The listing builds one solid part. Answer for the finished solid, in the listing's coordinates (mm). Face numbers are marked on the shaded views. Coordinates: 2 decimals unless noted, no trailing zeros. Write each loop counter-clockwise with the first axis right and the second up, starting at its lowest first coordinate (ties: lowest second). Pieces come first, ordered by that corner, then holes.
from build123d import *

# Parameters (mm, degrees)
CROQUIS1_W              = 7
CROQUIS1_H              = 18.3
SALIENTE_EXTRUIR1_DEPTH = 2.6
CORTAR_EXTRUIR2_DEPTH   = 10
REDONDEO1_R             = 1.5


with BuildPart() as part:
    # Croquis1 → Saliente-Extruir1 (new body)
    with BuildSketch(Plane(origin=(0, 0, 0), x_dir=(1, 0, 0), z_dir=(0, 1, 0))):
        Rectangle(CROQUIS1_W, CROQUIS1_H)
    extrude(amount=SALIENTE_EXTRUIR1_DEPTH)

    # Croquis2 → Cortar-Extruir2 (cut)
    with BuildSketch(Plane(origin=(0, 2.6, 0), x_dir=(1, 0, 0), z_dir=(0, 1, 0))):
        with BuildLine():
            ThreePointArc((3.25, 3.725), (3.426776695, 3.651776695), (3.5, 3.475))
            Line((3.5, 3.475), (3.5, 6.225))
            ThreePointArc((3.5, 6.225), (3.426776695, 6.048223305), (3.25, 5.975))
            Line((3.25, 5.975), (2.767072698, 5.975))
            ThreePointArc((2.767072698, 5.975), (2.651546276, 6.003293785), (2.562169292, 6.081770833))
            ThreePointArc((2.562169292, 6.081770833), (-1.35, 4.85), (2.562169292, 3.618229167))
            ThreePointArc((2.562169292, 3.618229167), (2.651546276, 3.696706215), (2.767072698, 3.725))
            Line((2.767072698, 3.725), (3.25, 3.725))
        make_face()
        with BuildLine():
            ThreePointArc((3.5, -3.475), (3.426776695, -3.651776695), (3.25, -3.725))
            Line((3.25, -3.725), (2.767072698, -3.725))
            ThreePointArc((2.767072698, -3.725), (2.651546276, -3.696706215), (2.562169292, -3.618229167))
            ThreePointArc((2.562169292, -3.618229167), (-1.35, -4.85), (2.562169292, -6.081770833))
            ThreePointArc((2.562169292, -6.081770833), (2.651546276, -6.003293785), (2.767072698, -5.975))
            Line((2.767072698, -5.975), (3.25, -5.975))
            ThreePointArc((3.25, -5.975), (3.426776695, -6.048223305), (3.5, -6.225))
            Line((3.5, -6.225), (3.5, -3.475))
        make_face()
    extrude(amount=-CORTAR_EXTRUIR2_DEPTH, mode=Mode.SUBTRACT)

    # Redondeo1
    redondeo1_edges = [part.edges().sort_by_distance(p)[0] for p in [
        (3.5, 1.3, 9.15),
        (3.5, 1.3, -9.15),
    ]]
    fillet(redondeo1_edges, radius=REDONDEO1_R)


solid = part.part
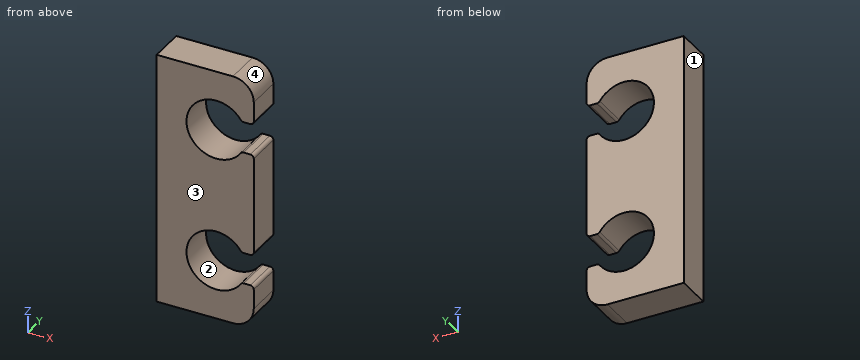
1. For a pull along X with two mould halves and no side action, classify the marked faces 1, 2, 3 and 4 as pulls with the +X half, pulls with the -X half, needs draft (parallel to the pull), parting line crosses it, or undercut.
Results found:
face 1: pulls with the -X half
face 2: undercut
face 3: needs draft
face 4: pulls with the +X half
2. Section B-B on y = 0.2 is taken. Give the vertices of the cut face in (x, z) (3 decimals).
Results found:
outline: (-3.5, -9.15) - (2, -9.15) arc R1.5 ccw to (3.5, -7.65) - (3.5, -6.225) arc R0.25 ccw to (3.25, -5.975) - (2.767, -5.975) arc R0.25 ccw to (2.562, -6.082) arc R2.15 cw (long way) to (2.562, -3.618) arc R0.25 ccw to (2.767, -3.725) - (3.25, -3.725) arc R0.25 ccw to (3.5, -3.475) - (3.5, 3.475) arc R0.25 ccw to (3.25, 3.725) - (2.767, 3.725) arc R0.25 ccw to (2.562, 3.618) arc R2.15 cw (long way) to (2.562, 6.082) arc R0.25 ccw to (2.767, 5.975) - (3.25, 5.975) arc R0.25 ccw to (3.5, 6.225) - (3.5, 7.65) arc R1.5 ccw to (2, 9.15) - (-3.5, 9.15) - close
3. Section A-A on x = 0.8 is taken. Give the vertices of the cut face in (y, z), then the cut area to 3 significant figures.
Results found:
outline: (0, -9.15) - (2.6, -9.15) - (2.6, -7) - (0, -7) - close; (0, -2.7) - (2.6, -2.7) - (2.6, 2.7) - (0, 2.7) - close; (0, 7) - (2.6, 7) - (2.6, 9.15) - (0, 9.15) - close
area: 25.2 mm2
4. Section D-D on x = 0 is taken. Give the vertices of the cut face in (y, z), then the cut area to 3 significant figures.
Results found:
outline: (0, -9.15) - (2.6, -9.15) - (2.6, -6.85) - (0, -6.85) - close; (0, -2.85) - (2.6, -2.85) - (2.6, 2.85) - (0, 2.85) - close; (0, 6.85) - (2.6, 6.85) - (2.6, 9.15) - (0, 9.15) - close
area: 26.8 mm2
5. Section C-C on z = -4.85 is taken. Give the vertices of the cut face in (x, y).
Results found:
outline: (-3.5, 0) - (-1.35, 0) - (-1.35, 2.6) - (-3.5, 2.6) - close
6. Find the intervals of material crossed by L1, parallel to Z at x = 0.8, y = 2; L2, parallel to Z at x = 2, y = 1.4; L3, parallel to X at y = 0.75, z = 4.85, in increasing order.
Results found:
L1: z = -9.15 to -7, -2.7 to 2.7, 7 to 9.15
L2: z = -9.15 to -6.63, -3.07 to 3.07, 6.63 to 9.15
L3: x = -3.5 to -1.35
